from build123d import *

# Parameters (mm, degrees)
BOSS_EXTRUDE2_DEPTH = 3
EXTRUDE_1_DEPTH     = 5
EXTRUDE_2_DEPTH     = 3


with BuildPart() as part:
    # Sketch3 → Boss-Extrude2 (new body)
    with BuildSketch(Plane.XY):
        with BuildLine():
            Line((-151, 81), (151, 81))
            ThreePointArc((151, 81), (158.071067812, 78.071067812), (161, 71))
            Line((161, 71), (161, -71))
            ThreePointArc((161, -71), (158.071067812, -78.071067812), (151, -81))
            Line((151, -81), (-151, -81))
            ThreePointArc((-151, -81), (-158.071067812, -78.071067812), (-161, -71))
            Line((-161, -71), (-161, 71))
            ThreePointArc((-161, 71), (-158.071067812, 78.071067812), (-151, 81))
        make_face()
    extrude(amount=-BOSS_EXTRUDE2_DEPTH)

    # Эскиз1 → Бобышка-Вытянуть1 (add)
    with BuildSketch(Plane(origin=(0, 0, -3), x_dir=(-1, 0, 0), z_dir=(0, 0, -1))):
        with BuildLine():
            Line((-151, -79), (151, -79))
            ThreePointArc((151, -79), (156.656854249, -76.656854249), (159, -71))
            Line((159, -71), (159, 71))
            ThreePointArc((159, 71), (156.656854249, 76.656854249), (151, 79))
            Line((151, 79), (-151, 79))
            ThreePointArc((-151, 79), (-156.656854249, 76.656854249), (-159, 71))
            Line((-159, 71), (-159, -71))
            ThreePointArc((-159, -71), (-156.656854249, -76.656854249), (-151, -79))
        make_face()
    extrude(amount=EXTRUDE_1_DEPTH)

    # Эскиз2 → Бобышка-Вытянуть2 (add)
    with BuildSketch(Plane.XY):
        with BuildLine():
            Line((162.5, 40), (162.5, 71))
            ThreePointArc((162.5, 71), (159.131727984, 79.131727984), (151, 82.5))
            Line((151, 82.5), (-151, 82.5))
            ThreePointArc((-151, 82.5), (-159.131727984, 79.131727984), (-162.5, 71))
            Line((-162.5, 71), (-162.5, -71))
            ThreePointArc((-162.5, -71), (-159.131727984, -79.131727984), (-151, -82.5))
            Line((-151, -82.5), (151, -82.5))
            ThreePointArc((151, -82.5), (159.131727984, -79.131727984), (162.5, -71))
            Line((162.5, -71), (162.5, -40))
            ThreePointArc((162.5, -40), (176, 0), (162.5, 40))
        make_face()
    extrude(amount=-EXTRUDE_2_DEPTH)


solid = part.part
Verification items for the finished model (mm, model axes). A direction names the side the tool comes from. Round coordinates to 2 decimals unless told otherwise and drop trailing zeros. Write each loop counter-clockwise with the first axis right and the second up, starting at its lowest first coordinate (ties: lowest second). Pieces come first, ordered by that corner, then holes.
(1) Material ranges on line 1 (X direction, y = -62.5, z = -5.75); line 2 (X direction, y = 68, z = -2.5); line 3 (Y direction, x = 36, z = -6.25), recorded low to high.
Returned:
line 1: x = -159 to 159
line 2: x = -162.5 to 162.5
line 3: y = -79 to 79
(2) Section check B-B (y = 65.5). Enter the section's corners in (x, z), plus the area to 4 significant figures.
Returned:
outline: (-162.5, -3) - (-159, -3) - (-159, -8) - (159, -8) - (159, -3) - (162.5, -3) - (162.5, 0) - (-162.5, 0) - close
area: 2,565 mm2
(3) Depth check by flat-ended pin: pin 1 Ø3 at (x, z) = (64, -7) entering from -Y; pin 2 Ø1.5 at (y, z) = (35.5, -5) entering from +X; pin 3 Ø3.5 at (y, z) = (-60, -1.5) entering from +X. Enter the tip coordinate at first touch or a pass-through.
Returned:
pin 1: stops at y = -79
pin 2: stops at x = 159
pin 3: stops at x = 162.5
(4) Section check A-A (z = -4.5). Enter the section's corners in (x, y).
Returned:
outline: (-159, -71) arc R8 ccw to (-151, -79) - (151, -79) arc R8 ccw to (159, -71) - (159, 71) arc R8 ccw to (151, 79) - (-151, 79) arc R8 ccw to (-159, 71) - close
(5) Access from +Z, -Z, +X, -X, +Y, -Y to the whole of each face (thin tool, end or side, straight path). Record for faces 1 (the cylindrical face through (156.594, 76.719, -5.465)), 2 (the cylindrical face through (-156.719, 76.594, -5.465)), 3 (the cylindrical face through (-156.594, -76.719, -5.465)).
Returned:
face 1: -Z, +X, +Y
face 2: -Z, -X, +Y
face 3: -Z, -X, -Y
